```python
from build123d import *

# Parameters (mm, degrees)
SKETCH1_R                = 1.5
SKETCH1_R_2              = 2.5
BOSS_EXTRUDE1_DEPTH      = 20
SKETCH2_W                = 8.1
SKETCH2_H                = 25
SKETCH2_W_2              = 3.1
SKETCH2_W_3              = 5.1
SKETCH2_H_2              = 20
CUT_EXTRUDE1_DEPTH       = 20
CUT_EXTRUDE1_DEPTH_BACK  = 20
CUT_EXTRUDE2_DEPTH       = 9
BOSS_EXTRUDE2_DEPTH      = 11.9
SKETCH5_R                = 3
BOSS_EXTRUDE3_DEPTH      = 3
CUT_EXTRUDE6_DEPTH       = 1
SKETCH13_R               = 2.5
CUT_EXTRUDE7_DEPTH       = 4
CUT_EXTRUDE5_START       = 5
CUT_EXTRUDE5_DEPTH       = 2
CUT_EXTRUDE8_REACH       = 22
SKETCH14_R               = 1.5
BOSS_EXTRUDE4_DEPTH      = 3
CUT_EXTRUDE9_DEPTH       = 3
SKETCH17_W               = 9
SKETCH17_H               = 3.569322199
CUT_EXTRUDE11_DEPTH      = 3
SKETCH18_W               = 5.770974844
SKETCH18_H               = 0.772936936
BOSS_EXTRUDE5_DEPTH      = 8.9
BOSS_EXTRUDE5_DEPTH_BACK = 1
SKETCH19_W               = 5.1
SKETCH19_H               = 16.397725614
CUT_EXTRUDE12_DEPTH      = 0.301495
SKETCH20_W               = 5
SKETCH20_H               = 12.419235667
CUT_EXTRUDE13_DEPTH      = 10


with BuildPart() as part:
    # Sketch1 → Boss-Extrude1 (new body)
    with BuildSketch(Plane(origin=(0, 0, 0), x_dir=(0, 0, -1), z_dir=(1, 0, 0))):
        with BuildLine():
            ThreePointArc((9.765353557, 20.116545894), (0, 32.270117322), (-9.765353557, 20.116545894))
            ThreePointArc((-9.765353557, 20.116545894), (-5.132645827, -18.047253777), (-7.88740095, -56.392382678))
            ThreePointArc((-7.88740095, -56.392382678), (0, -65.729882678), (7.88740095, -56.392382678))
            ThreePointArc((7.88740095, -56.392382678), (5.132645827, -18.047253777), (9.765353557, 20.116545894))
        make_face()
        with Locations((0, 22.270117322)):
            Circle(SKETCH1_R, mode=Mode.SUBTRACT)
        with Locations((0, -57.729882678)):
            Circle(SKETCH1_R_2, mode=Mode.SUBTRACT)
    extrude(amount=BOSS_EXTRUDE1_DEPTH)

    # Sketch2 → Cut-Extrude1 (cut, two sides)
    with BuildSketch(Plane.XY) as cut_extrude1_sk:
        with Locations((4.05, -53.229882678)):
            Rectangle(SKETCH2_W, SKETCH2_H)
        with Locations((18.45, -53.229882678)):
            Rectangle(SKETCH2_W_2, SKETCH2_H)
        with Locations((5.55, 22.270117322)):
            Rectangle(SKETCH2_W_3, SKETCH2_H_2)
    extrude(amount=CUT_EXTRUDE1_DEPTH, mode=Mode.SUBTRACT)
    extrude(cut_extrude1_sk.sketch, amount=-CUT_EXTRUDE1_DEPTH_BACK, mode=Mode.SUBTRACT)

    # Sketch3 → Cut-Extrude2 (cut)
    with BuildSketch(Plane.ZY.offset(-8.1)):
        with BuildLine():
            Line((8.5, 22.270117322), (8.5, 40.909533312))
            Line((8.5, 40.909533312), (-17.52872033, 40.909533312))
            Line((-17.52872033, 40.909533312), (-17.52872033, 13.770117322))
            Line((-17.52872033, 13.770117322), (0, 13.770117322))
            ThreePointArc((0, 13.770117322), (6.01040764, 16.259709682), (8.5, 22.270117322))
        make_face()
    extrude(amount=-CUT_EXTRUDE2_DEPTH, mode=Mode.SUBTRACT)

    # Sketch4 → Boss-Extrude2 (add, through all)
    with BuildSketch(Plane.ZY.offset(-8.1)):
        Polygon((8.5, 27.537944199), (8.283796844, 12.741558936), (10.283796844, 12.741558936), (10.283796844, 27.537944199), align=None)
    extrude(amount=-BOSS_EXTRUDE2_DEPTH)

    # Sketch5 → Boss-Extrude3 (add)
    with BuildSketch(Plane.ZY.offset(-8.1)):
        with BuildLine():
            Line((8.145156861, 11.968622), (8.447845456, 23.968622))
            Line((8.447845456, 23.968622), (9.854698466, 23.968622))
            Line((9.854698466, 23.968622), (14.022421388, 23.968622))
            ThreePointArc((14.022421388, 23.968622), (20.022421388, 17.968622), (14.022421388, 11.968622))
            Line((14.022421388, 11.968622), (8.145156861, 11.968622))
        make_face()
        with Locations((14.022421388, 17.968622)):
            Circle(SKETCH5_R, mode=Mode.SUBTRACT)
    extrude(amount=-BOSS_EXTRUDE3_DEPTH)

    # Sketch12 → Cut-Extrude6 (cut)
    with BuildSketch(Plane(origin=(11.1, 0, 0), x_dir=(0, 0, -1), z_dir=(1, 0, 0))):
        Polygon((-15.022421388, 13.968622), (-15.022421388, 12.968622), (-13.022421388, 12.968622), (-13.022421388, 13.968622), (-13.022421388, 15.140194875), (-14.022421388, 15.140194875), (-15.022421388, 15.140194875), align=None)
    extrude(amount=-CUT_EXTRUDE6_DEPTH, mode=Mode.SUBTRACT)

    # Sketch13 → Cut-Extrude7 (cut)
    with BuildSketch(Plane.ZY.offset(-17.1)):
        with Locations((0, 22.270117322)):
            Circle(SKETCH13_R)
    extrude(amount=-CUT_EXTRUDE7_DEPTH, mode=Mode.SUBTRACT)

    # Sketch10 → Cut-Extrude5 (cut)
    with BuildSketch(Plane.ZY.offset(-17.1).offset(CUT_EXTRUDE5_START)):
        with BuildLine():
            Line((8.283796844, 12.741558936), (6.251490054, 12.741558936))
            ThreePointArc((6.251490054, 12.741558936), (3.274825885, -13.914467314), (3.856000489, -40.729882678))
            Line((3.856000489, -40.729882678), (5.863867222, -40.729882678))
            Line((5.863867222, -40.729882678), (7.833024243, -40.729882678))
            Line((7.833024243, -40.729882678), (8.283796844, 12.741558936))
        make_face()
    extrude(amount=CUT_EXTRUDE5_DEPTH, mode=Mode.SUBTRACT)

    # Sketch14 → Cut-Extrude8 (cut, up to next)
    with BuildSketch(Plane.ZY, mode=Mode.PRIVATE) as cut_extrude8_sk1:
        with Locations((7.532575614, 18.331804915)):
            Circle(SKETCH14_R)
    cut_extrude8_tool1 = extrude(cut_extrude8_sk1.sketch, amount=-CUT_EXTRUDE8_REACH, mode=Mode.PRIVATE) & part.part
    add(cut_extrude8_tool1.solids().sort_by_distance((0, 18.331805, 7.532576))[0], mode=Mode.SUBTRACT)

    # Sketch15 → Boss-Extrude4 (add)
    with BuildSketch(Plane.ZY):
        Polygon((10, 22.270117322), (10, 11.968622), (8.145156861, 11.968622), (7.595672539, 11.968622), align=None)
    extrude(amount=-BOSS_EXTRUDE4_DEPTH)

    # Sketch16 → Cut-Extrude9 (cut)
    with BuildSketch(Plane(origin=(20, 0, 0), x_dir=(0, 0, -1), z_dir=(1, 0, 0))):
        with BuildLine():
            Line((-10.283796844, 23.968622), (-9.854698466, 23.968622))
            ThreePointArc((-9.854698466, 23.968622), (-9.349264901, 25.818531871), (-8.5, 27.537944199))
            Line((-8.5, 27.537944199), (-10.283796844, 27.537944199))
            Line((-10.283796844, 27.537944199), (-10.283796844, 23.968622))
        make_face()
    extrude(amount=-CUT_EXTRUDE9_DEPTH, mode=Mode.SUBTRACT)

    # Sketch17 → Cut-Extrude11 (cut)
    with BuildSketch(Plane.XY.offset(10.283796844)):
        with Locations((12.6, 25.7532831)):
            Rectangle(SKETCH17_W, SKETCH17_H)
    extrude(amount=-CUT_EXTRUDE11_DEPTH, mode=Mode.SUBTRACT)

    # Sketch18 → Boss-Extrude5 (add, two sides)
    with BuildSketch(Plane(origin=(11.1, 0, 0), x_dir=(0, 0, -1), z_dir=(1, 0, 0))) as boss_extrude5_sk:
        with Locations((-7.398309422, 12.355090468)):
            Rectangle(SKETCH18_W, SKETCH18_H)
    extrude(amount=BOSS_EXTRUDE5_DEPTH)
    extrude(boss_extrude5_sk.sketch, amount=-BOSS_EXTRUDE5_DEPTH_BACK)

    # Sketch19 → Cut-Extrude12 (cut)
    with BuildSketch(Plane(origin=(0, 12.270117322, 0), x_dir=(1, 0, 0), z_dir=(0, 1, 0))):
        with Locations((5.55, 0)):
            Rectangle(SKETCH19_W, SKETCH19_H)
    extrude(amount=-CUT_EXTRUDE12_DEPTH, mode=Mode.SUBTRACT)

    # Sketch20 → Cut-Extrude13 (cut)
    with BuildSketch(Plane.ZY.offset(-17.1)):
        with Locations((0, 28.479735156)):
            Rectangle(SKETCH20_W, SKETCH20_H)
    extrude(amount=-CUT_EXTRUDE13_DEPTH, mode=Mode.SUBTRACT)


solid = part.part
```
Geometry: final body of the model. Coordinates: model frame, mm. A direction names the side the tool comes from. Round coordinates to 2 decimals unless told otherwise and drop trailing zeros. Write each loop counter-clockwise with the first axis right and the second up, starting at its lowest first coordinate (ties: lowest second). Pieces come first, ordered by that corner, then holes. Notation, with made-up numbers: (38, 11.5) -> (78, 11.5) arc R27 cw to (78, 34.5) -> close; hole circle Ø2 at (-21, 43.25). An arc over 180 degrees is marked (long way). Use CSV: the item, a comma, the result in double quotes. Start each with the question number.
Q1. Pull-direction query (X, two-part tool) for faces 1 (the face through (0, 4, 0)), 2 (the face through (11, 23.969, 10)), 3 (the face through (1.479, 23.535, -0.806)), 4 (the face through (17.1, 21, -2.4)); classes: pulls with the +X half, pulls with the -X half, needs draft (parallel to the pull), parting line crosses it, or undercut.
Q2. Section D-D (y = -32). Return loops of the section in (x, z).
Q3. Section A-A (z = 16). Return loops of the section in (x, y), plus the area to 3 significant figures.
Q4. Section C-C (x = 1.5). Return loops of the section in (y, z).
Q5. Section B-B (y = -1). Return loops of the section in (x, z).
Q6. Line query: L1, parallel to Y at x = 2.1, z = 0; L2, parallel to Y at x = 16, z = 9.5; L3, parallel to Y at x = 7.75, z = 1. Output: solid intervals per line, ascending.
Q7. Reachability of faces 5 (the face through (1.479, 16.867, 7.207)), 6 (the face through (1, 17, 10)), 7 (the face through (1, 11.969, 9)), 8 (the face through (13, 13.77, -4)) from +Z, -Z, +X, -X, +Y, -Y: full face, straight path, thin tool, end or side. Return the list, or none.
Q8. First-contact query: pin 1 Ø0.5 at (x, y) = (10.5, 13.5) entering from +Z; pin 2 Ø10 at (x, y) = (13, -47.5) entering from -Z; pin 3 Ø6 at (x, y) = (13, -47) entering from -Z; pin 4 Ø2.5 at (y, z) = (22.27, 0) entering from +X. Flat tips, straight axial feed; report the tip coordinate or a pass-through.
Result sheet:
1,face 1,"pulls with the -X half"
1,face 2,"undercut"
1,face 3,"needs draft"
1,face 4,"undercut"
2,outline,"(0, -5.28) -> (20, -5.28) -> (20, 5.28) -> (12.1, 5.28) -> (12.1, 3.28) -> (10.1, 3.28) -> (10.1, 5.28) -> (0, 5.28) -> close"
3,outline,"(8.1, 12.3) -> (11.1, 12.3) -> (11.1, 15.71) -> (8.1, 15.71) -> close; (8.1, 20.22) -> (11.1, 20.22) -> (11.1, 23.63) -> (8.1, 23.63) -> close"
3,area,"20.5 mm²"
4,outline,"(-40.73, -5.86) arc R200 cw to (20.12, -9.77) arc R10 ccw (long way) to (22.27, 10) -> (11.97, 10) -> (11.97, 8.15) arc R200 cw to (-40.73, 5.86) -> close; hole circle Ø3 at (18.33, 7.53); hole circle Ø3 at (22.27, 0)"
5,outline,"(0, -6.28) -> (20, -6.28) -> (20, 6.28) -> (12.1, 6.28) -> (12.1, 4.27) -> (10.1, 4.27) -> (10.1, 6.28) -> (0, 6.28) -> close"
6,L1,"-40.73 to 20.77, 23.77 to 32.27"
6,L2,"11.97 to 23.97"
6,L3,"-40.73 to 11.97"
7,face 5,"-X"
7,face 6,"+Z, -X, +Y, -Y"
7,face 7,"+Z, +X, -X, -Y"
7,face 8,"-Z, +Y"
8,pin 1,"z = 18.29"
8,pin 2,"z = -7.27"
8,pin 3,"z = -6.91"
8,pin 4,"through"
